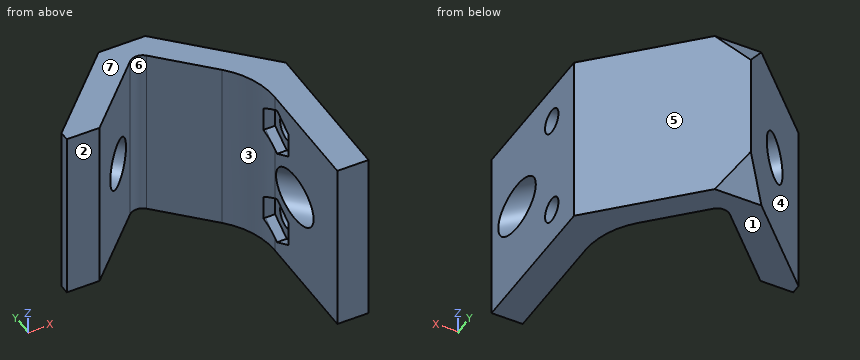
```python
from build123d import *

# Parameters (mm, degrees)
EXTRUDE_505_DEPTH      = 22.5
SKETCH_2_R             = 3.125
SMA_DEPTH              = 42.358123054
SKETCH_3_R             = 1.575
CUT_EXTRUDE_957_DEPTH  = 41.923198727
CUT_EXTRUDE_2_DEPTH    = 1.25
CUT_EXTRUDE_1673_DEPTH = 42.700155069
FILLET_1_R             = 10
FILLET_2_R             = 1.5


with BuildPart() as part:
    # Sketch 1 → Extrude 505 (new body)
    with BuildSketch(Plane.XY):
        Polygon((14.253048327, 0), (14.253048327, -19.446194078), (10.253048327, -19.446194078), (10.253048327, -0.596194078), (0, 9.656854249), (-9.656854249, 0), (-13.859292911, 0), (-13.859292911, 1.242283553), (-0.424264069, 14.677312396), align=None)
    extrude(amount=EXTRUDE_505_DEPTH)

    # Sketch 2 → SMA接口 (cut, through all)
    with BuildSketch(Plane(origin=(-7.550788232, 7.550788232, 0), x_dir=(0, 0, 1), z_dir=(-0.7071067811865486, 0.7071067811865465, 0))):
        with Locations(Location((11.25, 0.578427125, 0), (0, 0, 270))):
            Circle(SKETCH_2_R)
    extrude(amount=-SMA_DEPTH, mode=Mode.SUBTRACT)

    # 草图3 → Cut-Extrude 957 (cut, through all)
    with BuildSketch(Plane(origin=(14.253048327, 0, 0), x_dir=(0, 0, -1), z_dir=(1, 0, 0))):
        with Locations(Location((-17.75, -5.25, 0), (0, 0, 90))):
            Circle(SKETCH_3_R)
        with Locations(Location((-4.75, -5.25, 0), (0, 0, 90))):
            Circle(SKETCH_3_R)
    extrude(amount=-CUT_EXTRUDE_957_DEPTH, mode=Mode.SUBTRACT)

    # 草图4 → 侧板接口-2 (cut)
    with BuildSketch(Plane.ZY.offset(-10.253048327)):
        Polygon((6.33771324, -8), (7.925426481, -5.25), (6.33771324, -2.5), (3.16228676, -2.5), (1.574573519, -5.25), (3.16228676, -8), align=None)
        Polygon((19.33771324, -8), (20.925426481, -5.25), (19.33771324, -2.5), (16.16228676, -2.5), (14.574573519, -5.25), (16.16228676, -8), align=None)
    extrude(amount=-CUT_EXTRUDE_2_DEPTH, mode=Mode.SUBTRACT)

    # 草图7 → Cut-Extrude 1673 (cut, through all)
    with BuildSketch(Plane(origin=(0, 8.084293197, -5.389528798), x_dir=(-1, 0, 0), z_dir=(0, -0.8320502943378436, 0.5547001962252295))):
        Polygon((0.424264069, -11.885734391), (-2.575735931, -6.477407477), (3.424264069, -6.477407477), align=None)
    cut_extrude_1673 = extrude(amount=-CUT_EXTRUDE_1673_DEPTH, mode=Mode.SUBTRACT)

    # 镜向1: Cut-Extrude 1673 across plane
    add(cut_extrude_1673.mirror(Plane.XY.offset(11.25)), mode=Mode.SUBTRACT)

    # 圆角1
    # the kernel refuses this fillet: 10 mm, written as the material it adds along each edge
    with BuildSketch(Plane(origin=(10.253048327, -0.596194078, 0), x_dir=(-0.7071067811865485, 0.7071067811865465, 0), z_dir=(0, 0, 1))) as fillet_1_piece_1_section:
        with BuildLine():
            CenterArc((FILLET_1_R * 0.414213562373, FILLET_1_R), FILLET_1_R, 225, 45)
            Line((-FILLET_1_R * 0.292893218813, FILLET_1_R * 0.292893218813), (0, 0))
            Line((0, 0), (FILLET_1_R * 0.414213562373, 0))
        make_face()
    fillet_1_piece_1 = extrude(amount=22.5, mode=Mode.PRIVATE)
    fillet_1_piece_1 = split(fillet_1_piece_1, bisect_by=Plane(origin=(9.571569557, -2.5, 2.084142207), z_dir=(0, 1, 0)), keep=Keep.TOP, mode=Mode.PRIVATE)
    add(fillet_1_piece_1)
    with BuildSketch(Plane(origin=(10.253048327, -0.596194078, 0), x_dir=(-0.7071067811865485, 0.7071067811865465, 0), z_dir=(0, 0, 1))) as fillet_1_piece_2_section:
        with BuildLine():
            CenterArc((FILLET_1_R * 0.414213562373, FILLET_1_R), FILLET_1_R, 225, 45)
            Line((-FILLET_1_R * 0.292893218813, FILLET_1_R * 0.292893218813), (0, 0))
            Line((0, 0), (FILLET_1_R * 0.414213562373, 0))
        make_face()
    fillet_1_piece_2 = extrude(amount=32.855339059, mode=Mode.PRIVATE)
    fillet_1_piece_2 = split(fillet_1_piece_2, bisect_by=Plane(origin=(10.174215165, -3.639691918, 2.504285324), z_dir=(0, 0.49999999999999994, -0.8660254037844389)), keep=Keep.TOP, mode=Mode.PRIVATE)
    add(fillet_1_piece_2)
    with BuildSketch(Plane(origin=(10.253048327, -0.596194078, -10.355339059), x_dir=(-0.7071067811865485, 0.7071067811865465, 0), z_dir=(0, 0, 1))) as fillet_1_piece_3_section:
        with BuildLine():
            CenterArc((FILLET_1_R * 0.414213562373, FILLET_1_R), FILLET_1_R, 225, 45)
            Line((-FILLET_1_R * 0.292893218813, FILLET_1_R * 0.292893218813), (0, 0))
            Line((0, 0), (FILLET_1_R * 0.414213562373, 0))
        make_face()
    fillet_1_piece_3 = extrude(amount=43.210678119, mode=Mode.PRIVATE)
    fillet_1_piece_3 = split(fillet_1_piece_3, bisect_by=Plane(origin=(10.175314786, -5.028011676, 14.702738538), z_dir=(0, 0.4999999999999995, -0.8660254037844389)), keep=Keep.TOP, mode=Mode.PRIVATE)
    fillet_1_piece_3 = split(fillet_1_piece_3, bisect_by=Plane(origin=(10.175314786, -5.028011676, 7.797261462), z_dir=(0, 0.49999999999999994, 0.8660254037844387)), keep=Keep.TOP, mode=Mode.PRIVATE)
    add(fillet_1_piece_3)
    with BuildSketch(Plane(origin=(10.253048327, -0.596194078, -10.355339059), x_dir=(-0.7071067811865485, 0.7071067811865465, 0), z_dir=(0, 0, 1))) as fillet_1_piece_4_section:
        with BuildLine():
            CenterArc((FILLET_1_R * 0.414213562373, FILLET_1_R), FILLET_1_R, 225, 45)
            Line((-FILLET_1_R * 0.292893218813, FILLET_1_R * 0.292893218813), (0, 0))
            Line((0, 0), (FILLET_1_R * 0.414213562373, 0))
        make_face()
    fillet_1_piece_4 = extrude(amount=32.855339059, mode=Mode.PRIVATE)
    fillet_1_piece_4 = split(fillet_1_piece_4, bisect_by=Plane(origin=(10.174215165, -3.639691918, 19.995714676), z_dir=(0, 0.4999999999999997, 0.8660254037844388)), keep=Keep.TOP, mode=Mode.PRIVATE)
    add(fillet_1_piece_4)

    # 圆角2
    fillet_2_edges = [part.edges().sort_by_distance(p)[0] for p in [
        (0, 9.656854249, 11.25),
    ]]
    fillet(fillet_2_edges, radius=FILLET_2_R)


solid = part.part
```
CAD build for the part. Positions are in the model's coordinates, mm. Face numbers are marked on the shaded views. A direction names the side the tool comes from. Coordinates: 2 decimals unless noted, no trailing zeros. Loops run counter-clockwise (first coordinate to the right, second up) from the corner with the lowest first, then second, coordinate; pieces in that order, holes last. Notation, with made-up numbers: (-2, 28.25) - (42, 28.25) arc R21 cw to (42, 67.25) - close; hole circle Ø6 at (36, -16). An arc over 180 degrees is marked (long way). Return JSON: item names as keys, results as strings.
1. Mould opens along X. For the marked faces 4, 5, 6 and 7 say: released by +X, released by -X, zero draft, split by the parting line, or undercut.
Result:
{"face 4": "released by -X", "face 5": "released by +X", "face 6": "undercut", "face 7": "zero draft"}
2. Band-saw the part on C-C (y = 7). State how many separate pieces and enclosed holes the cut face has, and give its area (3 significant figures).
Result:
{"separate pieces": "3", "enclosed holes": "0", "area": "195 mm2"}
3. Band-saw the part on D-D (z = 2.75). Give the cut face in (x, y), and give its area (3 significant figures).
Result:
{"outline": "(-13.86, 0) - (-9.66, 0) - (-1.06, 8.6) arc R1.5 cw to (1.06, 8.6) - (7.32, 2.33) arc R10 cw to (10.14, -3.21) - (11.5, -3.21) - (11.5, -7.29) - (10.25, -7.29) - (10.25, -19.45) - (14.25, -19.45) - (14.25, 0) - (0.74, 13.51) - (-1.59, 13.51) - (-13.86, 1.24) - close", "area": "195 mm2"}
4. Band-saw the part on B-B (x = 0). Give the cut face in (y, z).
Result:
{"outline": "(9.04, 0) - (11.68, 0) - (14.25, 3.86) - (14.25, 18.64) - (11.68, 22.5) - (9.04, 22.5) - close"}
5. 3-axis set-ups, long thin cutter, end or side, ignore diameter. For the marked faces 1, 2 and 3: which of +Z, -Z, +X, -X, +Y, -Y reach the whole face in a straight line?
Result:
{"face 1": "-Z, +X, -X, +Y, -Y", "face 2": "+Z, -Z, -X, -Y", "face 3": "+Z, -Z, -Y"}
6. Band-saw the part on A-A (z = 9.75). Give the cut face in (x, y), and give its area (3 significant figures).
Result:
{"outline": "(-13.86, 0) - (-9.66, 0) - (-6.36, 3.3) - (-9.08, 6.02) - (-13.86, 1.24) - close; (-5.2, 9.9) - (-2.48, 7.18) - (-1.06, 8.6) arc R1.5 cw to (1.06, 8.6) - (7.32, 2.33) arc R10 cw to (10.25, -4.74) - (10.25, -5.56) - (14.25, -9.56) - (14.25, 0) - (-0.42, 14.68) - close; (10.25, -19.45) - (14.25, -19.45) - (14.25, -17.31) - (10.25, -13.31) - close", "area": "150 mm2"}
7. Drop flat-ended pins along their axis: pin 1 (12 mm diameter, centred on x = -8, z = 13.5, fed in from -Y); pin 2 (3 mm diameter, centred on x = -9, z = 3, fed in from +Y); pin 3 (1.4 mm diameter, centred on x = 10.5, z = 18, fed in from +Y). Give the stop position or say it passes through.
Result:
{"pin 1": "stops at y = 0", "pin 2": "stops at y = 7.6", "pin 3": "stops at y = 4.45"}
8. Probe L1, parallel to Z at x = 13.35, y = -5.25 (3 decimals); L2, parallel to X at y = 2.5, z = 6; L3, parallel to X at y = -13.5, z = 8.75. List the from-to ranges inside material, lowest first. Write a range as from..to.
Result:
{"L1": "z = 0..3.175, 6.325..16.175, 19.325..22.5", "L2": "x = -12.6..-7.16, 7.16..11.75", "L3": "x = 10.25..11.67"}
